For this review, use the dimensioned drawing (mm, ordinates from the lowest corner) and the shaded views. A direction names the side the tool comes from. Coordinates: 2 decimals unless noted, no trailing zeros. Order: outer loops, then holes, each group sorted by start corner. A loop starts at its lowest first (then second) coordinate and runs counter-clockwise, first axis right, second up. Notation, with made-up numbers: M 63,74.5 L 85,74.5 A31 ccw 85,103.5 Z; hole C -19.75,73.5 d9. An arc over 180 degrees is marked long. Use CSV: the item, a comma, the result in double quotes.
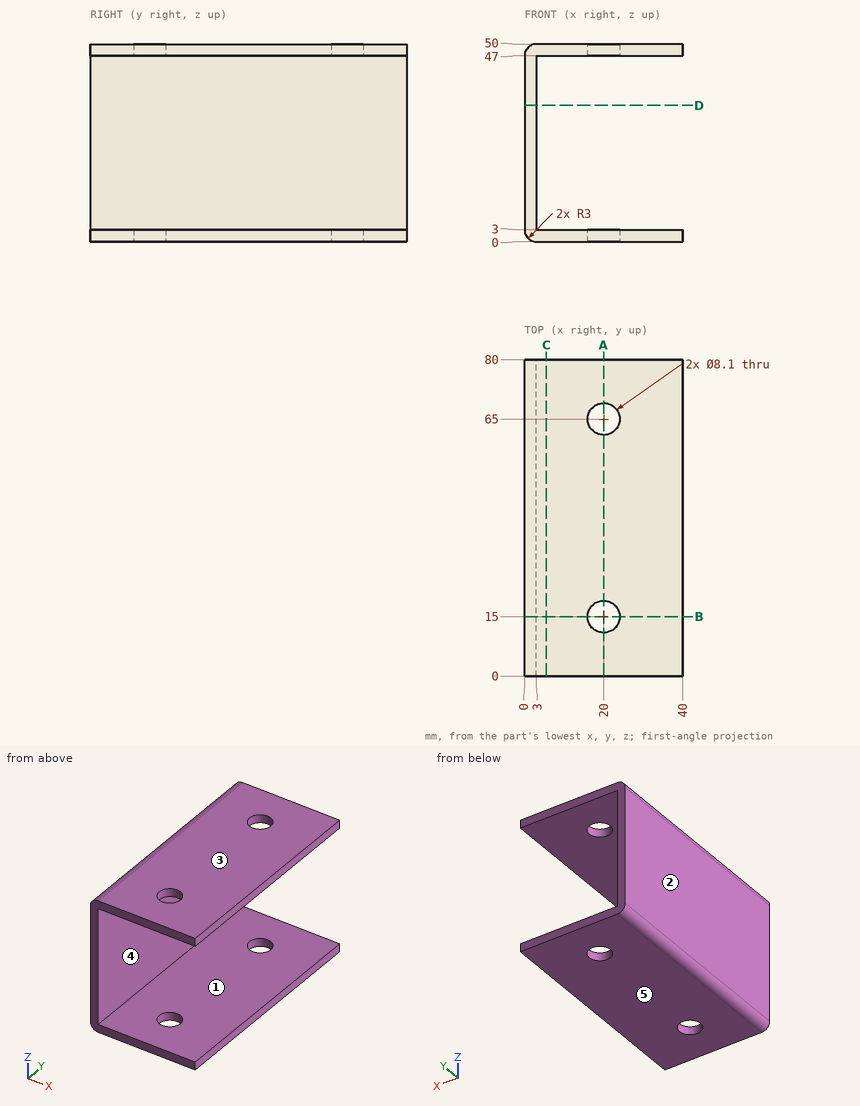
Item 1: Add section B-B on y = 15. State the section outline as (x, z) points.
Solutions:
outline,"M 0,3 A3 ccw 3,0 L 15.95,0 L 15.95,3 L 3,3 L 3,47 L 15.95,47 L 15.95,50 L 3,50 A3 ccw 0,47 Z; M 24.05,0 L 40,0 L 40,3 L 24.05,3 Z; M 24.05,47 L 40,47 L 40,50 L 24.05,50 Z"
Item 2: Clearance check with flat-ended pins moving along their axes: pin 1 Ø6.5 at (x, y) = (20, 65) entering from +Z; pin 2 Ø5 at (y, z) = (50.5, 37.5) entering from +X. State where each tip first meets the part, or that it passes through.
Solutions:
pin 1,"through"
pin 2,"x = 3"
Item 3: Add section A-A on x = 20. State the section outline as (y, z) points, and give its area (3 significant figures).
Solutions:
outline,"M 0,0 L 10.95,0 L 10.95,3 L 0,3 Z; M 0,47 L 10.95,47 L 10.95,50 L 0,50 Z; M 19.05,0 L 60.95,0 L 60.95,3 L 19.05,3 Z; M 19.05,47 L 60.95,47 L 60.95,50 L 19.05,50 Z; M 69.05,0 L 80,0 L 80,3 L 69.05,3 Z; M 69.05,47 L 80,47 L 80,50 L 69.05,50 Z"
area,"383 mm^2"
Item 4: To check wall thickness, follow line 1 along Z through (x, y) = (6.5, 62.5); line 2 along Y through (x, z) = (20, 48); line 3 along X through (y, z) = (42.5, 12). State the ranges of each line that lie inside material, in increasing order. Write a range as [from, to].
Solutions:
line 1,"[0, 3], [47, 50]"
line 2,"[0, 10.95], [19.05, 60.95], [69.05, 80]"
line 3,"[0, 3]"
Item 5: Draft analysis for pull direction Z (two halves, no side actions). For the marked faces 3, 4 and 5, state which applies: released by +Z, released by -Z, zero draft, split by the parting line, or undercut.
Solutions:
face 3,"released by +Z"
face 4,"undercut"
face 5,"released by -Z"
Item 6: Add section D-D on z = 34.5. State the section outline as (x, y) points, and give its area (3 significant figures).
Solutions:
outline,"M 0,0 L 3,0 L 3,80 L 0,80 Z"
area,"240 mm^2"
Item 7: For the marked faces 1 and 2, list the 3-axis set-ups (+Z, -Z, +X, -X, +Y, -Y) from which the entire face can be reached by the end or side of a thin tool; tool diameter is ignored.
Solutions:
face 1,"+X, +Y, -Y"
face 2,"+Z, -Z, -X, +Y, -Y"
Item 8: Add section C-C on x = 5.5. State the section outline as (y, z) points, and give its area (3 significant figures).
Solutions:
outline,"M 0,0 L 80,0 L 80,3 L 0,3 Z; M 0,47 L 80,47 L 80,50 L 0,50 Z"
area,"480 mm^2"
